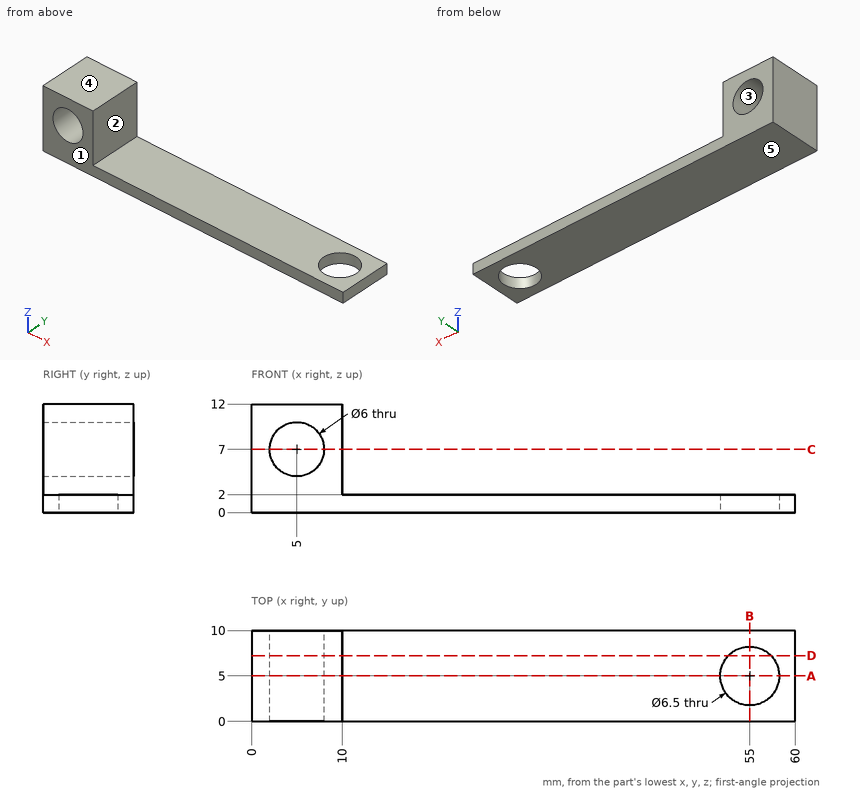
Source: three-view drawing plus pictorial views. Frame: mm from the lowest corner of the part. A direction names the side the tool comes from. Coordinates: 2 decimals unless noted, no trailing zeros. Write each loop counter-clockwise with the first axis right and the second up, starting at its lowest first coordinate (ties: lowest second). Pieces come first, ordered by that corner, then holes. Notation, with made-up numbers: (-33.5, -18) - (-5.5, -18) arc R24 cw to (-5.5, -3) - close; hole circle Ø5 at (-13.75, 28). An arc over 180 degrees is marked (long way). Answer as a JSON object with one key per item and string values.
Q1. Set-up query: the marked faces 1 and 2. Return all of +Z, -Z, +X, -X, +Y, -Y with unobstructed straight access to the full face (end or side cutting, diameter ignored); none if empty.
Ans:
{"face 1": "+Z, -Z, +X, -X, -Y", "face 2": "+Z, +X, +Y, -Y"}
Q2. Draft query along Z for the marked faces 3, 4 and 5. Return one class per face: released by +Z, released by -Z, zero draft, split by the parting line, or undercut.
Ans:
{"face 3": "undercut", "face 4": "released by +Z", "face 5": "released by -Z"}
Q3. First-contact query: pin 1 Ø3 at (x, y) = (35.5, 6.5) entering from +Z; pin 2 Ø5 at (y, z) = (2.5, 9) entering from +X. Flat tips, straight axial feed; report the tip coordinate or a pass-through.
Ans:
{"pin 1": "stops at z = 2", "pin 2": "stops at x = 10"}
Q4. Material intervals for line 1 (Y direction, x = 55, z = 0.85); line 2 (X direction, y = 5, z = 0.65); line 3 (Z direction, x = 5, y = 4.75), sorted ascending. Write a range as [from, to].
Ans:
{"line 1": "y = [0, 1.75], [8.25, 10]", "line 2": "x = [0, 51.75], [58.25, 60]", "line 3": "z = [0, 4], [10, 12]"}
Q5. Section query D-D, the plane y = 7.25. Output: boundary loops of the cut face in (x, z).
Ans:
{"outline": "(0, 0) - (52.65, 0) - (52.65, 2) - (10, 2) - (10, 12) - (0, 12) - close; (57.35, 0) - (60, 0) - (60, 2) - (57.35, 2) - close; hole circle Ø6 at (5, 7)"}
Q6. Section query C-C, the plane z = 7. Output: boundary loops of the cut face in (x, y).
Ans:
{"outline": "(0, 0) - (2, 0) - (2, 10) - (0, 10) - close; (8, 0) - (10, 0) - (10, 10) - (8, 10) - close"}
Q7. Section query A-A, the plane y = 5. Output: boundary loops of the cut face in (x, z).
Ans:
{"outline": "(0, 0) - (51.75, 0) - (51.75, 2) - (10, 2) - (10, 12) - (0, 12) - close; (58.25, 0) - (60, 0) - (60, 2) - (58.25, 2) - close; hole circle Ø6 at (5, 7)"}
Q8. Section query B-B, the plane x = 55. Output: boundary loops of the cut face in (y, z), plus the area to 3 significant figures.
Ans:
{"outline": "(0, 0) - (1.75, 0) - (1.75, 2) - (0, 2) - close; (8.25, 0) - (10, 0) - (10, 2) - (8.25, 2) - close", "area": "7.00 mm2"}
